Check sheet for the modelled part. Datum: model origin and axes. Units: mm. Round coordinates to 2 decimals unless told otherwise and drop trailing zeros. Loops run counter-clockwise (first coordinate to the right, second up) from the corner with the lowest first, then second, coordinate; pieces in that order, holes last. Notation, with made-up numbers: M -11.5,1.25 L 35.5,1.25 A30 cw 35.5,39.25 Z; hole C -4,12 d6. An arc over 180 degrees is marked long. One line per question, with ' | ' between items. Start each with the question number.
(1) Section check B-B (x = -56.5). Record the boundary of the cut face in (y, z), and give its area (3 significant figures).
(2) Section check D-D (x = -158). Record the boundary of the cut face in (y, z).
(3) Go/stop test with flat-tipped pins: P1, Ø9.5, axis at x = -25.5, y = -11, coming from the +Z side; P2, Ø5.5, axis at y = -19, z = 4.5, coming from the +X side; P3, Ø1.5, axis at x = -55.5, y = -20, coming from the -Z side. Record where each tip stops, or that it passes through.
(4) Section check A-A (z = 86.5). Record the boundary of the cut face in (x, y), and give its area (3 significant figures).
(5) Section check C-C (z = -18). Record the boundary of the cut face in (x, y).
(6) Thickness scan on probe 1 along X at (y, z) = (-19.5, -19.5); probe 2 along X at (y, z) = (-15.5, 97.5); probe 3 along Z at (x, y) = (-66, -9.25). Record the ranges inside material, lowest first. Write a range as [from, to].
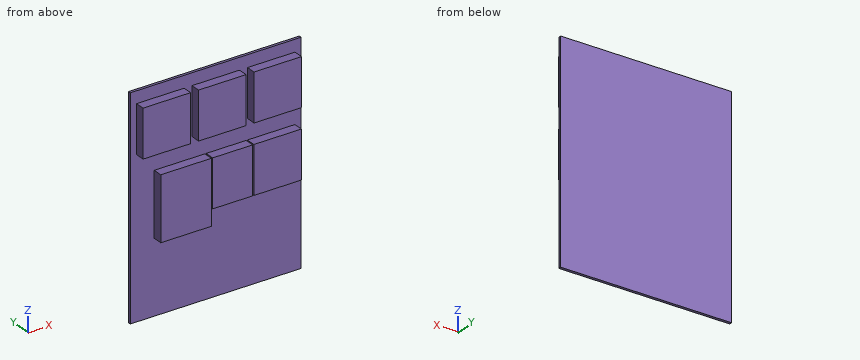
```python
from build123d import *

# Parameters (mm, degrees)
F0_W     = 342.9
F0_H     = 431.8
F1_DEPTH = 5.334
F2_W     = 95.25
F2_H     = 95.25
F2_W_2   = 80.27
F3_DEPTH = 19.05


# Not quite as in the source:
# - a feature names something its author has since deleted; it is built from what else it names


with BuildPart() as f1:
    # F0 (on Front) → F1 (new body)
    with BuildSketch(Plane.XZ):
        with Locations((-26.3048716933, -22.2786769863)):
            Rectangle(F0_W, F0_H)
    extrude(amount=F1_DEPTH)

    # F2 (on face) → F3 (join)
    with BuildSketch(Plane.XZ.offset(5.334)):
        with Locations((-137.4298716933, 121.9963230137)):
            Rectangle(F2_W, F2_H)
        with Locations((-26.1798716933, 121.9963230137)):
            Rectangle(F2_W, F2_H)
        with Locations((85.0701283067, 121.9963230137)):
            Rectangle(F2_W, F2_H)
        Polygon((-48.1548716933, 34.3713230137), (-149.7548716933, 34.3713230137), (-149.7548716933, -92.6286769863), (-48.1548716933, -92.6286769863), (-48.1548716933, -60.8786769863), align=None)
        with Locations((-5.4798716933, -13.2536769863)):
            Rectangle(F2_W_2, F2_H)
        with Locations((84.8201283067, -13.2536769863)):
            Rectangle(F2_W, F2_H)
    extrude(amount=F3_DEPTH)


solid = f1.part
```
The answers:
1) outline: M -24.38,-92.63 L -5.33,-92.63 L -5.33,-238.18 L 0,-238.18 L 0,193.62 L -5.33,193.62 L -5.33,169.62 L -24.38,169.62 L -24.38,74.37 L -5.33,74.37 L -5.33,34.37 L -24.38,34.37 Z | area: 6,540 mm²
2) outline: M -24.38,74.37 L -5.33,74.37 L -5.33,-238.18 L 0,-238.18 L 0,193.62 L -5.33,193.62 L -5.33,169.62 L -24.38,169.62 Z
3) P1: z = 169.62 | P2: x = 132.45 | P3: z = -92.63
4) outline: M -197.75,-5.33 L -185.05,-5.33 L -185.05,-24.38 L -89.8,-24.38 L -89.8,-5.33 L -73.8,-5.33 L -73.8,-24.38 L 21.45,-24.38 L 21.45,-5.33 L 37.45,-5.33 L 37.45,-24.38 L 132.7,-24.38 L 132.7,-5.33 L 145.15,-5.33 L 145.15,0 L -197.75,0 Z | area: 7,270 mm²
5) outline: M -197.75,-5.33 L -149.75,-5.33 L -149.75,-24.38 L -48.15,-24.38 L -48.15,-5.33 L -45.61,-5.33 L -45.61,-24.38 L 34.66,-24.38 L 34.66,-5.33 L 37.2,-5.33 L 37.2,-24.38 L 132.45,-24.38 L 132.45,-5.33 L 145.15,-5.33 L 145.15,0 L -197.75,0 Z
6) probe 1: [-149.75, -48.15], [-45.61, 34.66], [37.2, 132.45] | probe 2: [-185.05, -89.8], [-73.8, 21.45], [37.45, 132.7] | probe 3: [-92.63, 34.37], [74.37, 169.62]
